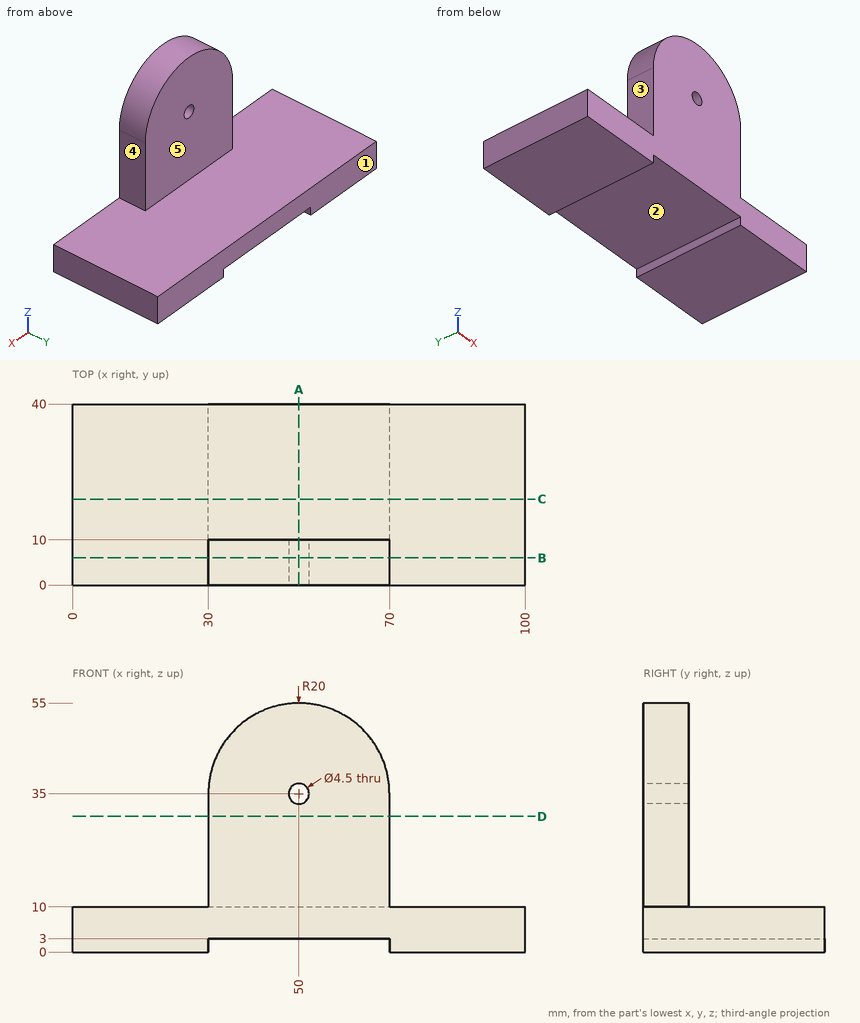
The figure shows three views and two pictorial views of one solid part (mm, origin at its lowest corner). Answer the questions. A direction names the side the tool comes from. Give positions to 0.01 mm unless a question says otherwise; leave off trailing zeros. Loops run counter-clockwise (first coordinate to the right, second up) from the corner with the lowest first, then second, coordinate; pieces in that order, holes last. Notation, with made-up numbers: (-21.5, 24.25) -> (19.5, 24.25) arc R19 ccw to (19.5, 35.25) -> close; hole circle Ø11 at (3, -19). An arc over 180 degrees is marked (long way). Use a Markdown table: item, result. Add a question column.
1. Find the intervals of material crossed by probe 1 along Z at (x, y) = (50, 4.5); probe 2 along Y at (x, z) = (55, 20), in increasing order.
2. Flat-ended cylindrical pins translate along their axes: pin 1 Ø6 at (y, z) = (9.5, 45.5) entering from +X; pin 2 Ø3 at (x, y) = (43, 14) entering from -Z; pin 3 Ø5 at (y, z) = (2.5, 20.5) entering from +X. Find the tip coordinate at first contact, or state that the pin passes through.
3. Section C-C on y = 19 is taken. Determine the outline of the cut face in (x, z).
4. For the marked faces 1, 2, 3, 4 and 5, determine the directions among +Z, -Z, +X, -X, +Y, -Y from which every point of the face is accessible in a straight line to the end or side of a thin tool.
5. Section A-A on x = 50 is taken. Determine the outline of the cut face in (y, z), and give its area (3 significant figures).
6. Section D-D on z = 30 is taken. Determine the outline of the cut face in (x, y).
7. Section B-B on y = 6 is taken. Determine the outline of the cut face in (x, z), and give its area (3 significant figures).
Results below:
| question | item | result |
|---|---|---|
| 1 | probe 1 | z = 3 to 32.75, 37.25 to 55 |
| 1 | probe 2 | y = 0 to 10 |
| 2 | pin 1 | stops at x = 68.54 |
| 2 | pin 2 | stops at z = 3 |
| 2 | pin 3 | stops at x = 70 |
| 3 | outline | (0, 0) -> (30, 0) -> (30, 3) -> (70, 3) -> (70, 0) -> (100, 0) -> (100, 10) -> (0, 10) -> close |
| 4 | face 1 | +Z, -Z, +X, -X, +Y |
| 4 | face 2 | -Z, +Y, -Y |
| 4 | face 3 | +Z, -X, +Y, -Y |
| 4 | face 4 | +Z, +X, +Y, -Y |
| 4 | face 5 | +Z, +X, -X, +Y |
| 5 | outline | (0, 3) -> (40, 3) -> (40, 10) -> (10, 10) -> (10, 32.75) -> (0, 32.75) -> close; (0, 37.25) -> (10, 37.25) -> (10, 55) -> (0, 55) -> close |
| 5 | area | 685 mm^2 |
| 6 | outline | (30, 0) -> (70, 0) -> (70, 10) -> (30, 10) -> close |
| 7 | outline | (0, 0) -> (30, 0) -> (30, 3) -> (70, 3) -> (70, 0) -> (100, 0) -> (100, 10) -> (70, 10) -> (70, 35) arc R20 ccw to (30, 35) -> (30, 10) -> (0, 10) -> close; hole circle Ø4.5 at (50, 35) |
| 7 | area | 2,490 mm^2 |
